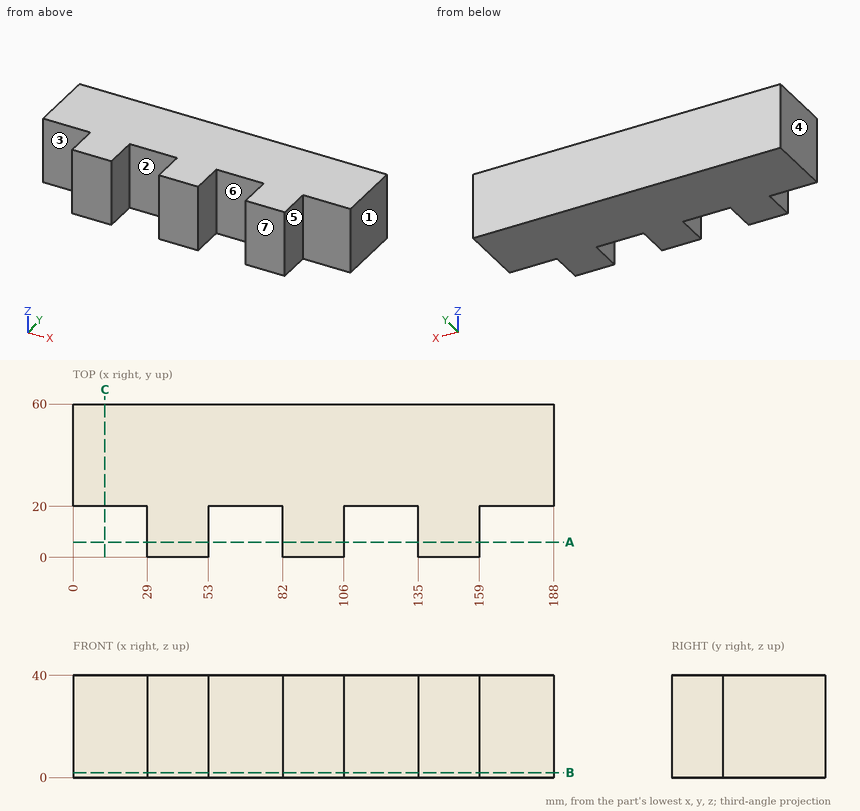
Study the drawing (mm; zero at the part's minimum x, y, z) and answer. A direction names the side the tool comes from. Give positions to 0.01 mm unless a question says otherwise; leave off trailing zeros. Loops run counter-clockwise (first coordinate to the right, second up) from the corner with the lowest first, then second, coordinate; pieces in that order, holes last. Notation, with made-up numbers: (63.25, 65.5) -> (101.25, 65.5) arc R15 ccw to (101.25, 77.5) -> close; hole circle Ø7 at (33.5, 31.5). An arc over 180 degrees is marked (long way). Write item = value, one per line. Start each with the question number.
(1) Find section C-C on x = 12.5. Give the vertices of the cut face in (y, z).
(2) Which of the six approach directions +Z, -Z, +X, -X, +Y, -Y give full straight-line access (tool end or side, diameter ignored) to the marked faces 5, 6 and 7?
(3) The mould has two halves that part along X. Classify the marked faces 1, 2, 3 and 4: +X half, -X half, draft (parallel to the pull), parting line (faces both ways), or undercut.
(4) Find the intervals of material crossed by probe 1 along X at (y, z) = (18, 8.5); probe 2 along Y at (x, z) = (58, 13), in increasing order. Write a range as from..to.
(5) Find section B-B on z = 2. Give the vertices of the cut face in (x, y).
(6) Find section A-A on y = 6. Give the vertices of the cut face in (x, z), and give its area (3 significant figures).
(7) Given pin 1 Ø6 at (y, z) = (10, 10.5) entering from +X; pin 2 Ø6 at (y, z) = (7.5, 16.5) entering from -X; pin 3 Ø8.5 at (x, z) = (115.5, 22.5) entering from -Y, each flat-ended and moving along its own axis, determine where each tip first touches the part or whether it passes through.
From the geometry:
q1.outline = (20, 0) -> (60, 0) -> (60, 40) -> (20, 40) -> close
q2.face_5 = +Z, -Z, +X, -Y
q2.face_6 = +Z, -Z, -Y
q2.face_7 = +Z, -Z, +X, -X, -Y
q3.face_1 = +X half
q3.face_2 = undercut
q3.face_3 = draft
q3.face_4 = -X half
q4.probe_1 = 29..53, 82..106, 135..159
q4.probe_2 = 20..60
q5.outline = (0, 20) -> (29, 20) -> (29, 0) -> (53, 0) -> (53, 20) -> (82, 20) -> (82, 0) -> (106, 0) -> (106, 20) -> (135, 20) -> (135, 0) -> (159, 0) -> (159, 20) -> (188, 20) -> (188, 60) -> (0, 60) -> close
q6.outline = (29, 0) -> (53, 0) -> (53, 40) -> (29, 40) -> close; (82, 0) -> (106, 0) -> (106, 40) -> (82, 40) -> close; (135, 0) -> (159, 0) -> (159, 40) -> (135, 40) -> close
q6.area = 2,880 mm^2
q7.pin_1 = 159
q7.pin_2 = 29
q7.pin_3 = 20
